Source: CAD feature listing. Evaluate the final solid. Frame: model axes, mm. Give positions to 0.01 mm unless a question says otherwise; leave off trailing zeros. Loops run counter-clockwise (first coordinate to the right, second up) from the corner with the lowest first, then second, coordinate; pieces in that order, holes last. Notation, with made-up numbers: M -15.75,-17.75 L 27.25,-17.75 A15 cw 27.25,3.25 Z; hole C 79.25,70.25 d7. An arc over 180 degrees is marked long. Answer in a Markdown table with one row per item.
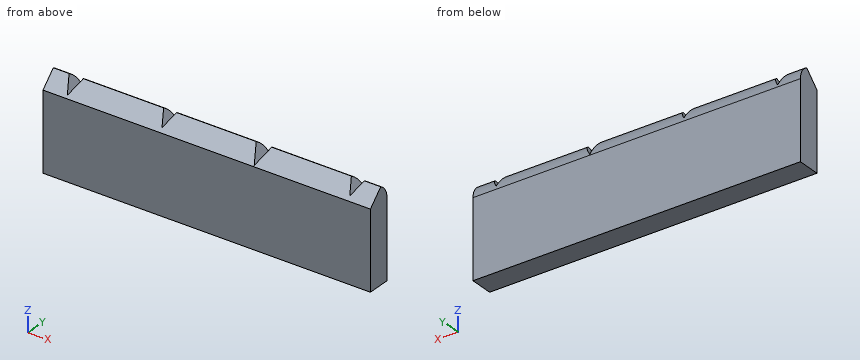
```python
from build123d import *

# Parameters (mm, degrees)
F0_W        = 36.322
F0_H        = 2.54
F1_DEPTH    = 10.414
F3_R        = 1.778
F4_T1_DEPTH = 45.4669047052
F5_DEPTH    = 25.4


# Not quite as in the source:
# - a fillet or chamfer that OpenCascade refuses, or shapes differently, is made with other operations: its cross-section is extruded or revolved along the edge and cut away or added


with BuildPart() as f1:
    # F0 (on Top) → F1 (new body)
    with BuildSketch(Plane.XY):
        with Locations((0, 1.27)):
            Rectangle(F0_W, F0_H)
    extrude(amount=F1_DEPTH)

    # F3
    f3_edges = [f1.edges().sort_by_distance(p)[0] for p in [
        (0, 2.54, 10.414),
    ]]
    fillet(f3_edges, radius=F3_R)

    # F4: chamfer of 1.778 on 1 edges, made by hand

    # F4_s2 → F4_t1 (cut)
    with BuildSketch(Plane.YZ.offset(-22.7334523526)):
        Polygon((1.778, 10.414), (0, 8.636), (0, 10.414), align=None)
    extrude(amount=F4_T1_DEPTH, mode=Mode.SUBTRACT)

    # F2 (on face) → F5 (cut)
    with BuildSketch(Plane.XZ):
        Polygon((-15.621, 8.8492954744), (-14.7176174209, 10.414), (-16.5243825791, 10.414), align=None)
        Polygon((-4.3769409051, 10.414), (-6.0370590949, 10.414), (-5.207, 8.9762954744), align=None)
        Polygon((6.1837060633, 10.414), (4.2302939367, 10.414), (5.207, 8.7222954744), align=None)
        Polygon((16.4510590949, 10.414), (14.7909409051, 10.414), (15.621, 8.9762954744), align=None)
    extrude(amount=-F5_DEPTH, mode=Mode.SUBTRACT)


solid = f1.part
```
Q1. Ray query, probe 1 along X at (y, z) = (1.95, 9.75); probe 2 along Y at (x, z) = (-17, 9.25); probe 3 along Z at (x, y) = (-2, 1.7). Return the intervals inside material, ascending. Write a range as from..to.
Values follow:
| item | result |
|---|---|
| probe 1 | -18.16..-16.14, -15.1..-5.65, -4.76..4.61, 5.8..15.17, 16.07..18.16 |
| probe 2 | 0.61..2.43 |
| probe 3 | 0..10.15 |
Q2. Contact query for a flat-ended pin moving along its axis: pin 1 Ø2 at (x, z) = (2, 7.5) entering from -Y. Output: stop coordinate, or through.
Values follow:
| item | result |
|---|---|
| pin 1 | y = 0 |
Q3. Section query A-A (x = 7). Output: boundary loops of the cut face in (y, z).
Values follow:
| item | result |
|---|---|
| outline | M 0,0 L 2.54,0 L 2.54,8.64 A1.78 ccw 1.58,10.22 L 0,8.64 Z |
Q4. Section query B-B (y = 2.1). Output: boundary loops of the cut face in (x, z).
Values follow:
| item | result |
|---|---|
| outline | M -18.16,0 L 18.16,0 L 18.16,9.81 L 16.1,9.81 L 15.62,8.98 L 15.14,9.81 L 5.83,9.81 L 5.21,8.72 L 4.58,9.81 L -4.73,9.81 L -5.21,8.98 L -5.69,9.81 L -15.07,9.81 L -15.62,8.85 L -16.17,9.81 L -18.16,9.81 Z |
